The figure shows three views and two pictorial views of one solid part (mm, origin at its lowest corner). Answer the questions. A direction names the side the tool comes from. Coordinates: 2 decimals unless noted, no trailing zeros. Write each loop counter-clockwise with the first axis right and the second up, starting at its lowest first coordinate (ties: lowest second). Pieces come first, ordered by that corner, then holes.
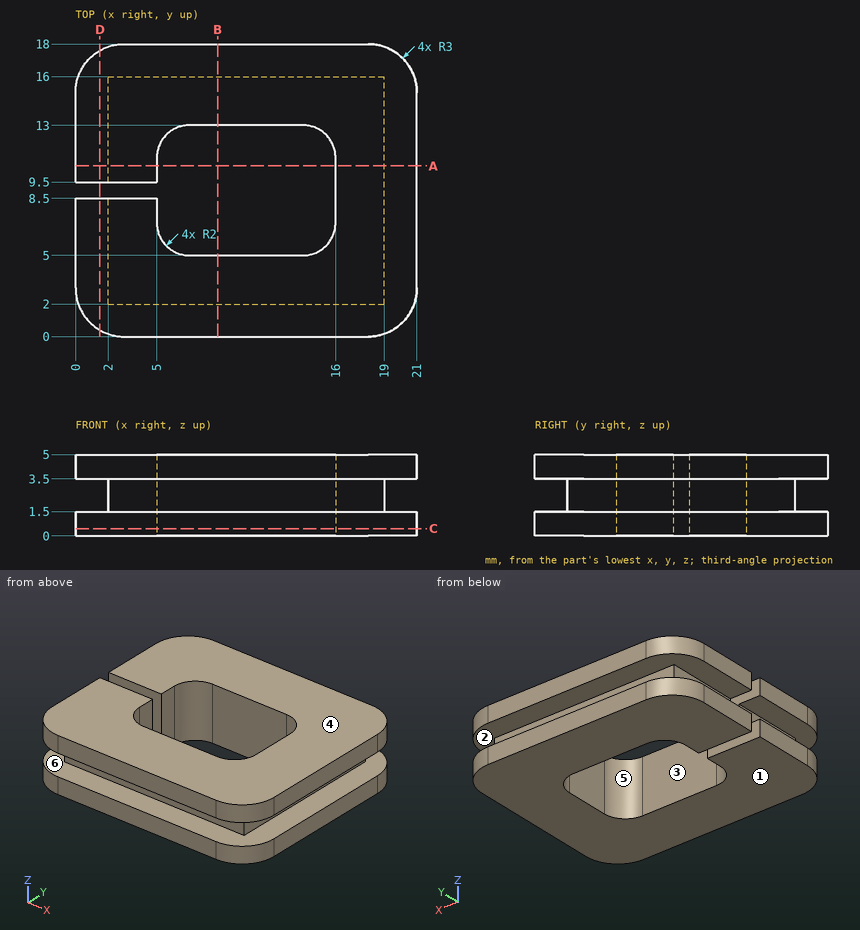
Q1. Given pin 1 (1.6 mm diameter, centred on x = 11, z = 2.5, fed in from -Y); pin 2 (0.6 mm diameter, centred on y = 11, z = 2.5, fed in from +X), each flat-ended and moving along its own axis, determine where each tip first touches the part or whether it passes through.
Answers below:
pin 1: stops at y = 2
pin 2: stops at x = 19
Q2. The part is cut by section D-D, the plane x = 1.5. Write down the section's boundary in (y, z), then the cut area to 3 significant figures.
Answers below:
outline: (0.4, 0) - (8.5, 0) - (8.5, 1.5) - (0.4, 1.5) - close; (0.4, 3.5) - (8.5, 3.5) - (8.5, 5) - (0.4, 5) - close; (9.5, 0) - (17.6, 0) - (17.6, 1.5) - (9.5, 1.5) - close; (9.5, 3.5) - (17.6, 3.5) - (17.6, 5) - (9.5, 5) - close
area: 48.6 mm2
Q3. The part is cut by section A-A, the plane y = 10.5. Write down the section's boundary in (x, z), then the cut area to 3 significant figures.
Answers below:
outline: (0, 0) - (5, 0) - (5, 5) - (0, 5) - (0, 3.5) - (2, 3.5) - (2, 1.5) - (0, 1.5) - close; (16, 0) - (21, 0) - (21, 1.5) - (19, 1.5) - (19, 3.5) - (21, 3.5) - (21, 5) - (16, 5) - close
area: 42.0 mm2
Q4. The part is cut by section C-C, the plane z = 0.45. Write down the section's boundary in (x, y).
Answers below:
outline: (0, 3) arc R3 ccw to (3, 0) - (18, 0) arc R3 ccw to (21, 3) - (21, 15) arc R3 ccw to (18, 18) - (3, 18) arc R3 ccw to (0, 15) - (0, 9.5) - (5, 9.5) - (5, 11) arc R2 cw to (7, 13) - (14, 13) arc R2 cw to (16, 11) - (16, 7) arc R2 cw to (14, 5) - (7, 5) arc R2 cw to (5, 7) - (5, 8.5) - (0, 8.5) - close
Q5. The part is cut by section B-B, the plane x = 8.75. Write down the section's boundary in (y, z), then the cut area to 3 significant figures.
Answers below:
outline: (0, 0) - (5, 0) - (5, 5) - (0, 5) - (0, 3.5) - (2, 3.5) - (2, 1.5) - (0, 1.5) - close; (13, 0) - (18, 0) - (18, 1.5) - (16, 1.5) - (16, 3.5) - (18, 3.5) - (18, 5) - (13, 5) - close
area: 42.0 mm2
Q6. Which of the six approach directions +Z, -Z, +X, -X, +Y, -Y give full straight-line access (tool end or side, diameter ignored) to the marked faces 1, 2 and 3?
Answers below:
face 1: -Z, +X, -X, +Y, -Y
face 2: none
face 3: +Z, -Z
Q7. Find the intervals of material crossed by probe 1 along Z at (x, y) = (19.25, 10); probe 2 along Y at (x, z) = (13, 1.2); probe 3 along Y at (x, z) = (3.75, 0.85), in increasing order.
Answers below:
probe 1: z = 0 to 1.5, 3.5 to 5
probe 2: y = 0 to 5, 13 to 18
probe 3: y = 0 to 8.5, 9.5 to 18
Q8. Determine the mould class of the marked faces 4, 5 and 6 for opening direction Z: released by +Z, released by -Z, zero draft, split by the parting line, or undercut.
Answers below:
face 4: released by +Z
face 5: zero draft
face 6: undercut
